Design review of the part built by this model. Coordinates are the model's own, in mm. Round coordinates to 2 decimals unless told otherwise and drop trailing zeros. Loops run counter-clockwise (first coordinate to the right, second up) from the corner with the lowest first, then second, coordinate; pieces in that order, holes last. Notation, with made-up numbers: (-4, 14) -> (33, 14) arc R11 ccw to (33, 25) -> close; hole circle Ø9 at (64, 81.5). An arc over 180 degrees is marked (long way). Use a Markdown table: item, result. Add a question column.
from build123d import *

# Parameters (mm, degrees)
BOSS_EXTRUDE1_DEPTH = 1.5
SKETCH1_3_W         = 5.23149294
SKETCH1_3_H         = 18.074674524
BOSS_EXTRUDE2_DEPTH = 2
SKETCH1_4_W         = 12.747878717
SKETCH1_4_H         = 3.806509515
BOSS_EXTRUDE3_DEPTH = 3.5
CHAMFER1_SIZE       = 1
CHAMFER2_SIZE       = 2.14222201
CHAMFER2_SIZE_2     = 1.5


with BuildPart() as part:
    # Sketch1 → Boss-Extrude1 (new, symmetric)
    with BuildSketch(Plane.XY):
        Polygon((0, 81.942442457), (0, 0), (5.23149294, 0), (5.23149294, 73.572714139), align=None)
    extrude(amount=BOSS_EXTRUDE1_DEPTH, both=True)



with BuildPart() as body_2:
    # Sketch1<3> → Boss-Extrude2 (new, symmetric)
    with BuildSketch(Plane.XY):
        with Locations((2.61574647, -12.843846777)):
            Rectangle(SKETCH1_3_W, SKETCH1_3_H)
    extrude(amount=BOSS_EXTRUDE2_DEPTH, both=True)


with BuildPart() as part_1:
    add(part.part)

    add(body_2.part)  # Boss-Extrude3 merges body 2
    # Sketch1<4> → Boss-Extrude3 (add, symmetric)
    with BuildSketch(Plane.XY):
        with Locations((2.615746471, -1.903254758)):
            Rectangle(SKETCH1_4_W, SKETCH1_4_H)
    extrude(amount=BOSS_EXTRUDE3_DEPTH, both=True)

    # Chamfer1
    chamfer1_edges = [part_1.edges().sort_by_distance(p)[0] for p in [
        (2.61574647, 0, 3.5),
        (8.989685829, 0, 0),
        (-3.758192888, -1.903254757, -3.5),
        (-3.758192888, 0, 0),
        (8.989685829, -1.903254757, 3.5),
        (-3.758192888, -1.903254757, 3.5),
        (2.61574647, 0, -3.5),
        (8.989685829, -1.903254757, -3.5),
        (0, -12.843846777, -2),
        (5.23149294, -12.843846777, 2),
        (0, -12.843846777, 2),
        (5.23149294, -12.843846777, -2),
    ]]
    chamfer(chamfer1_edges, length=CHAMFER1_SIZE)

    # Chamfer2
    # the kernel refuses this chamfer: 2.14222201, 1.5 mm, written as the material it takes off along each edge
    with BuildSketch(Plane(origin=(5.23149294, 0, 1.5), x_dir=(-0.99975333476413, 0, 0.022209674198456916), z_dir=(0, 1, 0))) as chamfer2_piece_1:
        Polygon((CHAMFER2_SIZE * 0.999753334817, -CHAMFER2_SIZE * 0.0222096741996), (-CHAMFER2_SIZE_2 * 0.0222096741985, -CHAMFER2_SIZE_2 * 0.999753334764), (0, 0), align=None)
    extrude(amount=79.105114369, mode=Mode.SUBTRACT)
    with BuildSketch(Plane(origin=(5.23149294, 0, -1.5), x_dir=(-0.99975333476413, 0, -0.022209674198456916), z_dir=(0, 1, 0))) as chamfer2_piece_2:
        Polygon((CHAMFER2_SIZE * 0.999753334817, CHAMFER2_SIZE * 0.0222096741996), (-CHAMFER2_SIZE_2 * 0.0222096741985, CHAMFER2_SIZE_2 * 0.999753334764), (0, 0), align=None)
    extrude(amount=79.105114369, mode=Mode.SUBTRACT)
    with BuildSketch(Plane(origin=(8.163825559, 68.881352106, 1.5), x_dir=(-0.8477703422928946, -0.5298982705204714, 0.02220967419845706), z_dir=(-0.530029010251303, 0.8479795093585836, 0))) as chamfer2_piece_3:
        Polygon((CHAMFER2_SIZE * 0.999753334817, -CHAMFER2_SIZE * 0.0222096741996), (-CHAMFER2_SIZE_2 * 0.0222096741985, -CHAMFER2_SIZE_2 * 0.999753334764), (0, 0), align=None)
    extrude(amount=20.935001598, mode=Mode.SUBTRACT)
    with BuildSketch(Plane(origin=(8.163825559, 68.881352106, -1.5), x_dir=(-0.8477703422928946, -0.5298982705204714, -0.02220967419845706), z_dir=(-0.530029010251303, 0.8479795093585836, 0))) as chamfer2_piece_4:
        Polygon((CHAMFER2_SIZE * 0.999753334817, CHAMFER2_SIZE * 0.0222096741996), (-CHAMFER2_SIZE_2 * 0.0222096741985, CHAMFER2_SIZE_2 * 0.999753334764), (0, 0), align=None)
    extrude(amount=20.935001598, mode=Mode.SUBTRACT)


solid = part_1.part
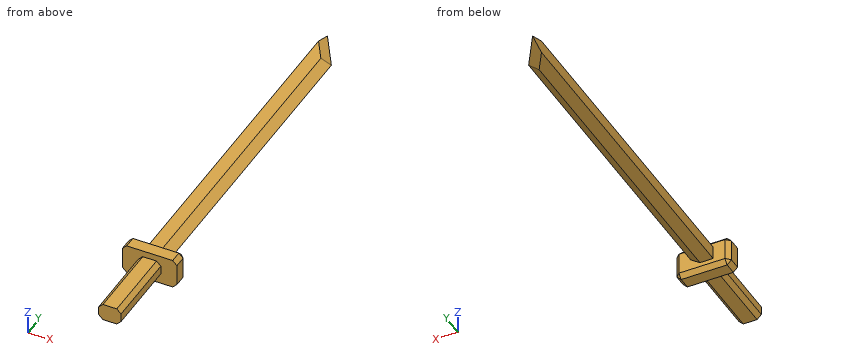
1. Consider section A-A on y = -8.5. State the section outline as (x, z) points, plus the area to 3 significant figures.
2. To check wall thickness, follow probe 1 along Y at (x, z) = (4.25, 0.75); probe 2 along Z at (x, y) = (1.5, 15.5); probe 3 along Y at (x, z) = (-1, 0.75). State the ranges of each line that lie inside material, in increasing order. Write a range as from..to.
3. Insertion check: P1, Ø2.5, axis at x = 2, y = 20, coming from the -Z side; P2, Ø0.9, axis at y = 50.5, z = -0.5, coming from the -X side; P3, Ø2, axis at y = -14.5, z = 0, coming from the +X side. Each pin has a flat end and moves straight along its axis. Give the tip position at first contact, or say it passes through.
4. Consider section C-C on y = 75.5. State the section outline as (x, z) points, plus the area to 3 significant figures.
5. Consider section B-B on y = 23.5. State the section outline as (x, z) points, plus the area to 3 significant figures.
Verdict:
| question | item | result |
|---|---|---|
| 1 | outline | (0, -1) -> (1, -2) -> (4.23, -2) -> (5.23, -1) -> (5.23, 1) -> (4.23, 2) -> (1, 2) -> (0, 1) -> close |
| 1 | area | 18.9 mm² |
| 2 | probe 1 | y = -21.88..0 |
| 2 | probe 2 | z = -1.5..1.5 |
| 2 | probe 3 | y = -3.81..0 |
| 3 | P1 | stops at z = -1.5 |
| 3 | P2 | stops at x = 0 |
| 3 | P3 | stops at x = 5.23 |
| 4 | outline | (0, -1.5) -> (1.5, -1.5) -> (4.03, 0) -> (1.5, 1.5) -> (0, 1.5) -> close |
| 4 | area | 8.29 mm² |
| 5 | outline | (0, -1.5) -> (3.09, -1.5) -> (5.23, 0) -> (3.09, 1.5) -> (0, 1.5) -> close |
| 5 | area | 12.5 mm² |
